The figure shows three views and two pictorial views of one solid part (mm, origin at its lowest corner). Answer the questions. A direction names the side the tool comes from. Coordinates: 2 decimals unless noted, no trailing zeros. Order: outer loops, then holes, each group sorted by start corner. A loop starts at its lowest first (then second) coordinate and runs counter-clockwise, first axis right, second up. Notation, with made-up numbers: (-39.75, 52) - (-12.75, 52) arc R24 ccw to (-12.75, 79) - close; hole circle Ø10 at (31, 35). An arc over 180 degrees is marked (long way). Answer as a JSON object with one key per item and string values. Group by question number.
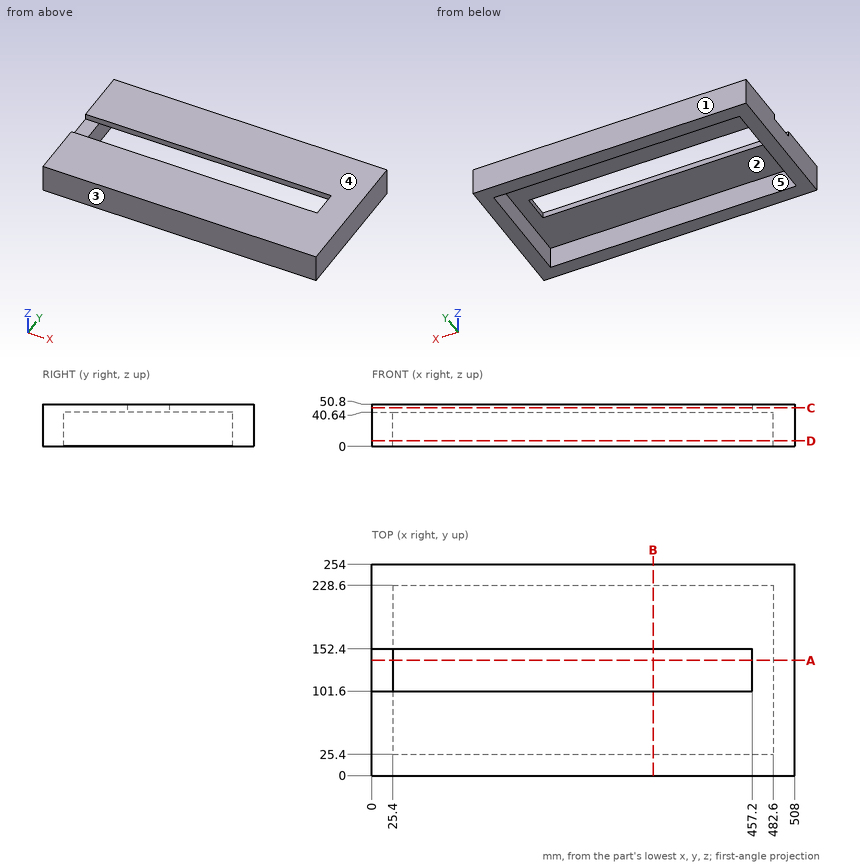
1. For the marked faces 1 and 2, determine the directions among +Z, -Z, +X, -X, +Y, -Y from which every point of the face is accessible in a straight line to the end or side of a thin tool.
2. A cutting plane is placed at B-B on x = 338. Write down the section's boundary in (y, z).
3. Straight lines are drawn through the part: L1, parallel to X at y = 42, z = 24.5; L2, parallel to Y at x = 75, z = 26; L3, parallel to Z at x = 290, y = 86. For each, find the intervals that lie inside material, in ascending order.
4. A cutting plane is placed at A-A on y = 138.5. Write down the section's boundary in (x, z).
5. A cutting plane is placed at C-C on z = 46. Write down the section's boundary in (x, y), and give its area (3 significant figures).
6. A cutting plane is placed at D-D on z = 6.5. Write down the section's boundary in (x, y).
7. For a pull along Y with two mould halves and no side action, classify the marked faces 3, 4 and 5 as pulls with the +Y half, pulls with the -Y half, needs draft (parallel to the pull), parting line crosses it, or undercut.
8. Given pin 1 (11 mm diameter, centred on y = 128, z = 48, fed in from -X); pin 2 (12 mm diameter, centred on x = 319.5, y = 101.5, fed in from -Z), each flat-ended and moving along its own axis, determine where each tip first touches the part or whether it passes through.
Derived:
{
 "1": {"face 1": "+Z, -Z, +X, -X, +Y", "face 2": "-Z"},
 "2": {"outline": "(0, 0) - (25.4, 0) - (25.4, 40.64) - (101.6, 40.64) - (101.6, 50.8) - (0, 50.8) - close; (152.4, 40.64) - (228.6, 40.64) - (228.6, 0) - (254, 0) - (254, 50.8) - (152.4, 50.8) - close"},
 "3": {"L1": "x = 0 to 25.4, 482.6 to 508", "L2": "y = 0 to 25.4, 228.6 to 254", "L3": "z = 40.64 to 50.8"},
 "4": {"outline": "(0, 0) - (25.4, 0) - (25.4, 40.64) - (0, 40.64) - close; (457.2, 40.64) - (482.6, 40.64) - (482.6, 0) - (508, 0) - (508, 50.8) - (457.2, 50.8) - close"},
 "5": {"outline": "(0, 0) - (508, 0) - (508, 254) - (0, 254) - (0, 152.4) - (457.2, 152.4) - (457.2, 101.6) - (0, 101.6) - close", "area": "106,000 mm2"},
 "6": {"outline": "(0, 0) - (508, 0) - (508, 254) - (0, 254) - close; hole (25.4, 25.4) - (482.6, 25.4) - (482.6, 228.6) - (25.4, 228.6) - close"},
 "7": {"face 3": "pulls with the -Y half", "face 4": "needs draft", "face 5": "undercut"},
 "8": {"pin 1": "stops at x = 457.2", "pin 2": "stops at z = 40.64"}
}
